Could you check a few things on this model? Use its own coordinates, in mm. A direction names the side the tool comes from. Coordinates: 2 decimals unless noted, no trailing zeros. Order: outer loops, then holes, each group sorted by start corner. A loop starts at its lowest first (then second) coordinate and runs counter-clockwise, first axis right, second up. Notation, with made-up numbers: M -38,17 L -29,17 A26 ccw -29,32 Z; hole C 3,-36.75 d7. An arc over 180 degrees is marked long. Write item = value, one per line. Start each with the question number.
from build123d import *

# Parameters (mm, degrees)
SKETCH1_W                      = 95
SKETCH1_H                      = 34
BOSS_EXTRUDE1_DEPTH            = 6.5
SKETCH2_W                      = 74
SKETCH2_H                      = 34
BOSS_EXTRUDE2_DEPTH            = 3.75
CBORE_FOR_M3_SHCS1_D           = 3.4
CBORE_FOR_M3_SHCS1_DEPTH       = 10.1
CBORE_FOR_M3_SHCS1_CBORE_D     = 6.5
CBORE_FOR_M3_SHCS1_CBORE_DEPTH = 3
CBORE_FOR_M3_SHCS1_TIP         = 1.021463052
CUT_EXTRUDE1_DEPTH             = 15.25
LPATTERN1_COUNT                = 4
LPATTERN1_PITCH                = 18


with BuildPart() as part:
    # Sketch1 → Boss-Extrude1 (new body)
    with BuildSketch(Plane.XY):
        Rectangle(SKETCH1_W, SKETCH1_H)
    extrude(amount=BOSS_EXTRUDE1_DEPTH)

    # Sketch2 → Boss-Extrude2 (add)
    with BuildSketch(Plane(origin=(0, 0, 0), x_dir=(-1, 0, 0), z_dir=(0, 0, -1))):
        Rectangle(SKETCH2_W, SKETCH2_H)
    extrude(amount=BOSS_EXTRUDE2_DEPTH)

    # CBORE for M3 SHCS1
    with Locations(Plane.XY.offset(6.5)):
        with Locations((-43.42, 10), (-43.42, -10), (43.42, 10), (43.42, -10)):
            CounterBoreHole(CBORE_FOR_M3_SHCS1_D / 2, CBORE_FOR_M3_SHCS1_CBORE_D / 2, CBORE_FOR_M3_SHCS1_CBORE_DEPTH, depth=CBORE_FOR_M3_SHCS1_DEPTH)
            with Locations((0, 0, -(CBORE_FOR_M3_SHCS1_DEPTH + CBORE_FOR_M3_SHCS1_TIP / 2))):  # 118° drill point
                Cone(0, CBORE_FOR_M3_SHCS1_D / 2, CBORE_FOR_M3_SHCS1_TIP, mode=Mode.SUBTRACT)

    # Sketch7 → Cut-Extrude1 (cut)
    with BuildSketch(Plane(origin=(33.5, 0, 0), x_dir=(0, 0, -1), z_dir=(1, 0, 0))):
        Polygon((-6.503383917, 8.006767833), (-3.756779362, 8.006767833), (-3.756779362, 9.003383917), (2.246616083, 9.003383917), (2.246616083, 7.503383917), (3.746616083, 7.503383917), (6.355468839, 7.503383917), (6.355468839, -12.746616083), (3.871124209, -12.746616083), (3.746616083, -12.746616083), (2.246616083, -12.746616083), (2.246616083, -14.496616083), (-3.756779362, -14.496616083), (-3.756779362, -9.25), (-6.503383917, -9.25), align=None)
    cut_extrude1 = extrude(amount=-CUT_EXTRUDE1_DEPTH, mode=Mode.SUBTRACT)

    # LPattern1: Cut-Extrude1 ×4
    with Locations(*[(-i * LPATTERN1_PITCH, 0, 0) for i in range(1, LPATTERN1_COUNT)]):
        add(cut_extrude1, mode=Mode.SUBTRACT)


solid = part.part
(1) For faces 1 (the flat face through (-28, 8.007, 5)), 2 (the flat face through (-1, 17, 1)), 3 (the flat face through (-28, -14.497, 1)), 4 (the flat face through (-1, 0, 6.5)), 5 (the flat face through (-28, -9.25, 5)), which set-ups out of +Z, -Z, +X, -X, +Y, -Y let a thin tool reach every point of the face, with its end or its side?
(2) Thinking about a two-plate mould opening in Z: for faces 6 (the flat face through (47.5, 0, 3)), 7 (the flat face through (8, -14, -2.247)), 8 (the flat face through (-42, -11.4, 3.5)), which applies, released by +Z, released by -Z, zero draft, split by the parting line, or undercut?
(3) Will these pins go through, and if not, where does the flat tip stop? P1, Ø8.5, axis at x = -44, y = -7, coming from the -Z side; P2, Ø3, axis at y = 3.5, z = -2, coming from the +X side; P3, Ø2, axis at x = 44.5, y = 9, coming from the +Z side.
(4) Imagine slicing it at D-D on x = 43.42. List the corners of the cut face in (y, z) for me, plus the area to 3 significant figures.
(5) Imagine slicing it at B-B on z = 1.25. Give the number of separate pieces and of enclosed holes in the cut face, plus the area to 3 significant figures.
(6) Please list where these lines run through material, in increasing order: probe 1 along Y at (x, z) = (-43.42, 2.05); probe 2 along Y at (x, z) = (43.42, 4.85); probe 3 along X at (y, z) = (-8, 1). Write a range as from..to.
(7) Imagine slicing it at A-A on x = -8. List the corners of the cut face in (y, z) for me.
(8) Imagine slicing it at C-C on y = 10. List the corners of the cut face in (x, z) for me, plus the area to 3 significant figures.
Response:
q1.face_1 = +Z
q1.face_2 = +Z, -Z, +X, -X, +Y
q1.face_3 = none
q1.face_4 = +Z, +X, -X, +Y, -Y
q1.face_5 = +Z, -Z
q2.face_6 = zero draft
q2.face_7 = undercut
q2.face_8 = released by +Z
q3.P1 = 0
q3.P2 = 37
q3.P3 = 3.5
q4.outline = M -17,0 L -11.7,0 L -11.7,3.5 L -13.25,3.5 L -13.25,6.5 L -17,6.5 Z; M -8.3,0 L 8.3,0 L 8.3,3.5 L 6.75,3.5 L 6.75,6.5 L -6.75,6.5 L -6.75,3.5 L -8.3,3.5 Z; M 11.7,0 L 17,0 L 17,6.5 L 13.25,6.5 L 13.25,3.5 L 11.7,3.5 Z
q4.area = 158 mm2
q5.separate_pieces = 1
q5.enclosed_holes = 8
q5.area = 1,760 mm2
q6.probe_1 = -17..-11.7, -8.3..8.3, 11.7..17
q6.probe_2 = -17..-13.25, -6.75..6.75, 13.25..17
q6.probe_3 = -47.5..-35.75, -20.5..-17.75, -2.5..0.25, 15.5..18.25, 33.5..47.5
q7.outline = M -17,-3.75 L -12.75,-3.75 L -12.75,-2.25 L -14.5,-2.25 L -14.5,3.76 L -9.25,3.76 L -9.25,6.5 L -17,6.5 Z; M 7.5,-3.75 L 17,-3.75 L 17,6.5 L 8.01,6.5 L 8.01,3.76 L 9,3.76 L 9,-2.25 L 7.5,-2.25 Z
q8.outline = M -47.5,0 L -45.12,0 L -45.12,3.5 L -46.67,3.5 L -46.67,6.5 L -47.5,6.5 Z; M -41.72,0 L -37,0 L -37,-3.75 L 37,-3.75 L 37,0 L 41.72,0 L 41.72,3.5 L 40.17,3.5 L 40.17,6.5 L -40.17,6.5 L -40.17,3.5 L -41.72,3.5 Z; M 45.12,0 L 47.5,0 L 47.5,6.5 L 46.67,6.5 L 46.67,3.5 L 45.12,3.5 Z
q8.area = 832 mm2
